Autodesk Inventor part; units mm, degrees
ref_plane "YZ Plane" through (0, 0, 0) normal (1, 0, 0) x (0, 1, 0)
ref_plane "XZ Plane" through (0, 0, 0) normal (0, 1, 0) x (-1, 0, 0)
ref_plane "XY Plane" through (0, 0, 0) normal (0, 0, 1) x (1, 0, 0)
sketch "Sketch1" plane through (0, 0, 0) normal (0, 1, 0) x (-1, 0, 0)
  line L0 (40, 57.5) -> (-40, 57.5)
  line L1 (-40, 57.5) -> (-40, -57.5)
  line L2 (-40, -57.5) -> (40, -57.5)
  line L3 (40, -57.5) -> (40, 57.5)
  point P0 (0, 0)
  point P1 (40, 0)
  point P2 (0, 57.5)
  dimension "d0" = 115
  dimension "d1" = 80
extrude "Extrusion1" add sketch "Sketch1" along normal blind 20
sketch "Sketch12" plane through (0, 0, 0) normal (0, -1, 0) x (1, 0, 0)
  line L0 (-40, 57.5) -> (-20, 57.5)
  line L1 (-20, 57.5) -> (-20, -57.5)
  line L2 (-20, -57.5) -> (-40, -57.5)
  line L3 (-40, -57.5) -> (-40, 57.5)
  line L4 (-40, -57.5) -> (-40, 57.5)
  line L5 (0, 100.8809) -> (0, -116.5773) construction
  line L6 (40, 57.5) -> (20, 57.5)
  line L7 (20, 57.5) -> (20, -57.5)
  line L8 (20, -57.5) -> (40, -57.5)
  line L9 (40, -57.5) -> (40, 57.5)
  point P0 (0, 0)
  point P1 (-40, 0)
  point P2 (0, 0)
  point P3 (-20, 0)
  dimension "d56" = 20
  dimension "d57" = 115
extrude "Extrusion11" add sketch "Sketch12" along normal blind 37.5
sketch "Sketch13" plane through (-40, 0, 57.5) normal (-1, 0, 0) x (0, 0, 1)
  line L0 (0, 0) -> (-115, 0)
  point P0 (-57.5, 0)
  point P1 (-22.5, -15)
  point P2 (-92.5, -15)
  point P3 (-57.5, -15)
  point P4 (-57.5, 0)
  dimension "d129" = 35
  dimension "d130" = 35
  dimension "d131" = 15
hole "Hole2" at (-40, -15, 35) at (-40, -15, -35) direction (1, 0, 0) diameter 20 end through all
hole "Hole3" at (-40, -15, 0) direction (1, 0, 0) diameter 15 end through all
sketch "Sketch19" plane through (0, 20, 0) normal (0, 1, 0) x (1, 0, 0)
  point P0 (0, 0)
  point P1 (25, 0)
  point P2 (-25, 0)
  dimension "d111" = 25
  dimension "d112" = 25
hole "Hole6" at (25, 20, 0) at (-25, 20, 0) direction (0, -1, 0) diameter 15 depth 15
fillet "Fillet19" radius 20 4 edges at (-30, -37.5, -57.5) (30, -37.5, -57.5) (30, -37.5, 57.5) (-30, -37.5, 57.5)
sketch "Sketch20" plane through (0, 20, 0) normal (0, 1, 0) x (1, 0, 0)
  line L0 (-27, -22.5) -> (27, -22.5)
  line L1 (27, -22.5) -> (27, -12.5)
  line L2 (27, -12.5) -> (-27, -12.5)
  line L3 (-27, -12.5) -> (-27, -22.5)
  line L4 (-40, 57.5) -> (-40, -57.5)
  line L5 (40, -57.5) -> (40, 57.5)
  line L6 (-40, -57.5) -> (40, -57.5)
  point P0 (0, 0)
  point P1 (0, -12.5)
  dimension "d122" = 10
  dimension "d151" = 45
  dimension "d152" = 54
extrude "Extrusion15" add sketch "Sketch20" along normal blind 44
sketch "Sketch21" plane through (-40, 20, 22.5) normal (0, 0, 1) x (1, 0, 0)
  circle A0 centre (40, 22) radius 7.5
  line L0 (20, -20) -> (60, -20)
  line L1 (13, 44) -> (67, 44)
  circle A1 centre (40, 22) radius 11
  point P0 (40, -20)
  point P1 (40, -20)
  point P2 (0, -20)
  point P3 (80, -20)
  point P4 (24.5, 37.5)
  point P5 (24.5, 6.5)
  point P6 (55.5, 6.5)
  point P7 (55.5, 37.5)
  dimension "d128" = 15
  dimension "d132" = 22
  dimension "d134" = 15.5
  dimension "d135" = 15.5
  dimension "d138" = 360
  dimension "d147" = 22
extrude "Extrusion16" cut sketch "Sketch21" against normal blind 50 contours A0
hole "Hole7" at (-15.5, 57.5, 22.5) at (-15.5, 26.5, 22.5) at (15.5, 26.5, 22.5) at (15.5, 57.5, 22.5) direction (0, 0, -1) diameter 5 depth 15
extrude "Extrusion17" cut sketch "Sketch21" against normal blind 2
sketch "Sketch24" plane through (0, 20, 0) normal (0, 1, 0) x (1, 0, 0)
  line L0 (-27, -22.5) -> (-22, -22.5)
  line L1 (-22, -22.5) -> (-22, -57.5)
  line L2 (-22, -57.5) -> (-27, -57.5)
  line L3 (-27, -57.5) -> (-27, -22.5)
  line L4 (-27, -22.5) -> (-27, -12.5)
  line L5 (27, -22.5) -> (-27, -22.5)
  line L6 (-40, -57.5) -> (40, -57.5)
  line L7 (22, -22.5) -> (27, -22.5)
  line L8 (27, -22.5) -> (27, -57.5)
  line L9 (27, -57.5) -> (22, -57.5)
  line L10 (22, -57.5) -> (22, -22.5)
  line L11 (27, -12.5) -> (27, -22.5)
  point P0 (0, 0)
  dimension "d155" = 5
  dimension "d156" = 5
extrude "Extrusion18" add sketch "Sketch24" along normal blind 44 contours L0 L1 L2 L3 | L5 L8 L6 L10
sketch "Sketch25" plane through (27, 20, 57.5) normal (1, 0, 0) x (0, 0, -1)
  line L0 (35, 44) -> (0, 0)
  line L1 (0, 44) -> (35, 44)
  line L2 (0, 44) -> (0, 0)
  line L3 (45, 0) -> (45, 44)
  point P0 (57.5, -20)
  dimension "d161" = 10
extrude "Extrusion19" cut sketch "Sketch25" against normal blind 100
properties part number "Y_Slider_Part_mit_Schrittmotor"
Work out the finished part from the listing and answer in its coordinate system (mm). A direction names the side the tool comes from. Round coordinates to 2 decimals unless told otherwise and drop trailing zeros. Write each loop counter-clockwise with the first axis right and the second up, starting at its lowest first coordinate (ties: lowest second). Pieces come first, ordered by that corner, then holes. Notation, with made-up numbers: (77.25, 0) - (114.25, 0) arc R11 ccw to (114.25, 9) - close; hole circle Ø2 at (46, -29.5). An arc over 180 degrees is marked (long way). Return JSON: item names as keys, results as strings. Group by question number.
Q1. For faces 4 (the flat face through (20, -23, 1)), 5 (the flat face through (-27, 37, 30)), 6 (the flat face through (-30, -37.5, 1)), 7 (the flat face through (22, 32, 32)), 8 (the flat face through (-25, 5, 0)), determine the directions among +Z, -Z, +X, -X, +Y, -Y from which every point of the face is accessible in a straight line to the end or side of a thin tool.
Q2. The part is cut by section C-C on x = 0. Write down the section's boundary in (y, z), then the cut area to 3 significant figures.
Q3. Find the intervals of material crossed by L1, parallel to Z at x = 28.5, y = -15; L2, parallel to X at y = 16, z = 0; L3, parallel to Y at x = -15.5, z = 18.75, in increasing order.
Q4. The part is cut by section B-B on y = -2.5. Write down the section's boundary in (x, z).
Q5. The mould has two halves that part along Y. Classify faces 1 (the cylindrical face through (30.1, -20.1, -5.5)), 2 (the flat face through (0, 64, 17)), 3 (the flat face through (-10, 37, 22.5)): released by +Y, released by -Y, zero draft, split by the parting line, or undercut.
Q6. The part is cut by section A-A on x = 25. Write down the section's boundary in (y, z).
Q7. The part is cut by section D-D on z = 9. Write down the section's boundary in (x, y).
Q8. Each of these flat-tipped pins is pushed along its axis until it touches: pin 1 Ø1 at (x, z) = (3, 46) entering from +Y; pin 2 Ø16 at (y, z) = (-15, 35) entering from +X; pin 3 Ø11 at (y, z) = (-12.5, -25.5) entering from -X; pin 4 Ø12 at (x, z) = (8, 44) entering from -Y. Where does it stop, or does it pass through?
Solved:
{
 "1": {"face 4": "+Z, -Z, -Y", "face 5": "+Z, -Z, -X, +Y", "face 6": "+Z, -Z, +X, -X, -Y", "face 7": "+Z, +Y", "face 8": "+Y"},
 "2": {"outline": "(0, -57.5) - (20, -57.5) - (20, 12.5) - (34.5, 12.5) - (34.5, 20.5) - (31, 20.5) - (31, 22.5) - (20, 22.5) - (20, 57.5) - (0, 57.5) - close; (49.5, 12.5) - (64, 12.5) - (64, 22.5) - (53, 22.5) - (53, 20.5) - (49.5, 20.5) - close", "area": "2,580 mm²"},
 "3": {"L1": "-57.5 to -45, -25 to -7.5, 7.5 to 25, 45 to 57.5", "L2": "-40 to -32.5, -17.5 to 17.5, 32.5 to 40", "L3": "0 to 24, 29 to 55, 60 to 64"},
 "4": {"outline": "(-40, -57.5) - (-20, -57.5) - (-20, 57.5) - (-40, 57.5) - close; (20, -57.5) - (40, -57.5) - (40, 57.5) - (20, 57.5) - close"},
 "5": {"face 1": "undercut", "face 2": "released by +Y", "face 3": "zero draft"},
 "6": {"outline": "(-37.5, -37.5) arc R20 ccw to (-17.5, -57.5) - (20, -57.5) - (20, -7.5) - (5, -7.5) - (5, 7.5) - (20, 7.5) - (20, 12.5) - (64, 12.5) - (64, 22.5) - (20, 57.5) - (-17.5, 57.5) arc R20 ccw to (-37.5, 37.5) - close; hole circle Ø20 at (-15, -35); hole circle Ø20 at (-15, 35); hole circle Ø15 at (-15, 0)"},
 "7": {"outline": "(-40, -37.5) - (-20, -37.5) - (-20, 0) - (20, 0) - (20, -37.5) - (40, -37.5) - (40, 20) - (-40, 20) - close"},
 "8": {"pin 1": "y = 20", "pin 2": "through", "pin 3": "x = -40", "pin 4": "y = 0"}
}
